```python
from build123d import *

# Parameters (mm, degrees)
BOSS_EXTRUDE1_DEPTH     = 12
SKETCH3_W               = 5
SKETCH3_H               = 20
BOSS_EXTRUDE2_DEPTH     = 12
CUT_EXTRUDE1_DEPTH      = 44.1052491
CUT_EXTRUDE1_DEPTH_BACK = 44.1052491
SKETCH4_W               = 17
SKETCH4_H               = 6
FILLET1_R               = 10


with BuildPart() as part:
    # Sketch2 → Boss-Extrude1 (new body)
    with BuildSketch(Plane(origin=(0, 0, 0), x_dir=(1, 0, 0), z_dir=(0, 1, 0))):
        Polygon((-6, -0.75), (-6, 11.25), (6, 11.25), (6, -0.75), (10, -0.75), (10, 16.25), (-10, 16.25), (-10, -0.75), align=None)
    extrude(amount=BOSS_EXTRUDE1_DEPTH)

    # Sketch3 → Boss-Extrude2 (add)
    with BuildSketch(Plane(origin=(0, 12, 0), x_dir=(1, 0, 0), z_dir=(0, 1, 0))):
        with Locations((0, 26.25)):
            Rectangle(SKETCH3_W, SKETCH3_H)
    extrude(amount=-BOSS_EXTRUDE2_DEPTH)

    # Sketch4 → Cut-Extrude1 (cut, two sides: drawn at the far end of the back side and taken through both)
    with BuildSketch(Plane(origin=(10, 0, 0), x_dir=(0, 0, -1), z_dir=(1, 0, 0)).offset(-CUT_EXTRUDE1_DEPTH_BACK)):
        with Locations((7.75, 9)):
            Rectangle(SKETCH4_W, SKETCH4_H)
    extrude(amount=CUT_EXTRUDE1_DEPTH + CUT_EXTRUDE1_DEPTH_BACK, mode=Mode.SUBTRACT)

    # Fillet1
    # the kernel refuses this fillet: 10 mm, written as the material it takes off along each edge
    with BuildSketch(Plane(origin=(25.412878475, 12, -16.25), x_dir=(0, -1, 0), z_dir=(-1, 0, 0))) as fillet1_piece_1:
        with BuildLine():
            CenterArc((10, -9.16515139), FILLET1_R, 113.578178478, 66.421821522)
            Line((0, -9.16515139), (-0.2, -9.16515139))
            Line((-0.2, -9.16515139), (-0.2, 0))
            Line((-0.2, 0), (0, 0.2))
            ThreePointArc((0, 0.2), (3, 0.2), (5.92, 0.183303028))
            Line((5.92, 0.183303028), (6, 0))
        make_face()
    extrude(amount=50.82575695, mode=Mode.SUBTRACT)


solid = part.part
```
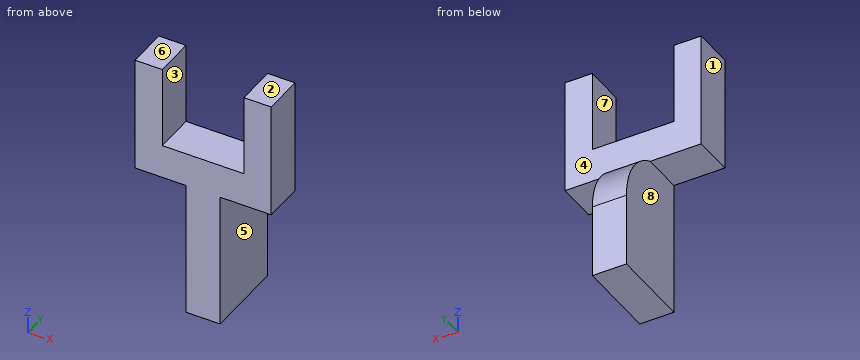
Verification items for the finished model (mm, model axes). Face numbers are marked on the shaded views. A direction names the side the tool comes from. Round coordinates to 2 decimals unless told otherwise and drop trailing zeros. Loops run counter-clockwise (first coordinate to the right, second up) from the corner with the lowest first, then second, coordinate; pieces in that order, holes last. Notation, with made-up numbers: (56.25, 50.25) -> (105.25, 50.25) arc R7 cw to (105.25, 55.25) -> close; hole circle Ø3 at (23.25, -20.5). An arc over 180 degrees is marked (long way). Answer as a JSON object with one key per item and string values.
Q1. Section check A-A (z = -1.5). Record the boundary of the cut face in (x, y).
Data:
{"outline": "(-10, 0) -> (-6, 0) -> (-6, 6) -> (-10, 6) -> close; (6, 0) -> (10, 0) -> (10, 6) -> (6, 6) -> close"}
Q2. Section check B-B (y = 3.25). Record the boundary of the cut face in (x, z).
Data:
{"outline": "(-10, -16.25) -> (-2.5, -16.25) -> (-2.5, -36.25) -> (2.5, -36.25) -> (2.5, -16.25) -> (10, -16.25) -> (10, 0.75) -> (6, 0.75) -> (6, -11.25) -> (-6, -11.25) -> (-6, 0.75) -> (-10, 0.75) -> close"}
Q3. Access from +Z, -Z, +X, -X, +Y, -Y to the whole of each face (thin tool, end or side, straight path). Record for the marked faces 4, 5, 6, 7 and 8.
Data:
{"face 4": "+Z, +X, -X, +Y", "face 5": "-Z, +X, +Y, -Y", "face 6": "+Z, +X, -X, +Y, -Y", "face 7": "+Z, +Y, -Y", "face 8": "-Z, -X, +Y, -Y"}
Q4. Go/stop test with flat-tipped pins: P1, Ø3, axis at x = 7, y = 5.5, coming from the -Z side; P2, Ø3, axis at x = -2.5, y = 2, coming from the +Z side; P3, Ø8.5, axis at x = 0, z = -8, coming from the +Y side. Record where each tip stops, or that it passes through.
Data:
{"P1": "stops at z = -16.25", "P2": "stops at z = -11.25", "P3": "stops at y = 6"}
Q5. Scan lines: line 1 (X direction, y = 5.75, z = -10); line 2 (X direction, y = 10, z = -26); line 3 (Z direction, x = 2, y = 3). Record each from-to range of solid material in increasing order. Write a range as from..to.
Data:
{"line 1": "x = -10..-6, 6..10", "line 2": "x = -2.5..2.5", "line 3": "z = -36.25..-11.25"}
Q6. Draft check along X on the marked faces 1, 2 and 3. Enter one of: pulls with the +X half, pulls with the -X half, needs draft (parallel to the pull), parting line crosses it, or undercut.
Data:
{"face 1": "pulls with the -X half", "face 2": "needs draft", "face 3": "undercut"}
Q7. Section check C-C (x = 1). Record the boundary of the cut face in (y, z).
Data:
{"outline": "(0, -36.25) -> (12, -36.25) -> (12, -25.42) arc R10 ccw to (6, -16.25) -> (6, -11.25) -> (0, -11.25) -> close"}
Q8. Section check D-D (z = -23). Record the boundary of the cut face in (x, y).
Data:
{"outline": "(-2.5, 0) -> (2.5, 0) -> (2.5, 11.7) -> (-2.5, 11.7) -> close"}
